from build123d import *

# Parameters (mm, degrees)
SHELL_3_T                 = 2
CUT_EXTRUDE_START         = 8.179460037
CUT_EXTRUDE_8_OUTLINE_W   = 19.681614291
CUT_EXTRUDE_8_OUTLINE_H   = 19.489043198
CUT_EXTRUDE_8_OUTLINE_W_2 = 22.765402734
CUT_EXTRUDE_8_OUTLINE_H_2 = 19.26138917
CUT_EXTRUDE_8_DEPTH       = 11.858295625
SKETCH_9_W                = 37.384578993
SKETCH_9_H                = 19.297136137
CUT_EXTRUDE_5_DEPTH       = 10
CUT_EXTRUDE_10_DEPTH      = 49


# Read off the part's stored shape, not the designer's step: the extrude step
with BuildPart() as part:
    # Sketch 5 → Loft 2 section 0
    with BuildSketch(Plane.XY):
        with BuildLine():
            Line((123.949416554, -29.058070489), (134.559011277, 0.091551442))
            Line((134.559011277, 0.091551442), (59.000774753, -54.400934133))
            Line((59.000774753, -54.400934133), (89.51414806, -54.400934133))
            Line((89.51414806, -54.400934133), (109.519294053, -29.058070489))
            Line((109.519294053, -29.058070489), (123.949416554, -29.058070489))
        make_face()
    # Sketch 2 → Loft 2 section 1
    with BuildSketch(Plane.XY.offset(-30)):
        with BuildLine():
            Line((134.559011277, 0.091551442), (123.949416554, -29.058070489))
            Line((123.949416554, -29.058070489), (109.519294053, -29.058070489))
            Line((109.519294053, -29.058070489), (89.51414806, -54.400934133))
            Line((89.51414806, -54.400934133), (59.000774753, -54.400934133))
            Line((59.000774753, -54.400934133), (134.559011277, 0.091551442))
        make_face()
    loft()

    # Shell 3
    shell_3_openings = [part.faces().sort_by_distance(p)[0] for p in [
        (99.793796859, -32.953132271, 0),
    ]]
    offset(amount=SHELL_3_T, openings=shell_3_openings, kind=Kind.INTERSECTION)

    # Cut-Extrude 8 outline → Cut-Extrude 8 (cut)
    with BuildSketch(Plane(origin=(45.99732156, -63.779004852, 0), x_dir=(0.8110731554347567, 0.5849447294686114, 0), z_dir=(0.5849447294686114, -0.8110731554347567, 0)).offset(CUT_EXTRUDE_START)):
        with Locations((87.31465052, -9.744521599)):
            Rectangle(CUT_EXTRUDE_8_OUTLINE_W, CUT_EXTRUDE_8_OUTLINE_H)
        with Locations((40.58343187, -9.630694585)):
            Rectangle(CUT_EXTRUDE_8_OUTLINE_W_2, CUT_EXTRUDE_8_OUTLINE_H_2)
    extrude(amount=CUT_EXTRUDE_8_DEPTH, mode=Mode.SUBTRACT)

    # Sketch 9 → Cut-Extrude 5 (cut)
    with BuildSketch(Plane(origin=(44.827432101, -62.156858541, 0), x_dir=(0.8110731554347567, 0.5849447294686114, 0), z_dir=(-0.5849447294686114, 0.8110731554347567, 0))):
        with Locations((72.683721601, 9.648568069)):
            Rectangle(SKETCH_9_W, SKETCH_9_H)
    extrude(amount=-CUT_EXTRUDE_5_DEPTH, mode=Mode.SUBTRACT)

    # Sketch 13 → Cut-Extrude 10 (cut)
    with BuildSketch(Plane.XY.offset(-30)):
        Polygon((78.963932985, -44.04826302), (81.023403307, -46.903885112), (89.476536517, -40.807498262), (87.417066196, -37.95187617), align=None)
        Polygon((103.880127445, -22.95550088), (118.225703578, -12.609493132), (121.093195937, -16.585503101), (106.747619804, -26.931510849), align=None)
    extrude(amount=-CUT_EXTRUDE_10_DEPTH, mode=Mode.SUBTRACT)


solid = part.part
Source: CAD feature listing. Evaluate the final solid. Frame: model axes, mm. A direction names the side the tool comes from. Give positions to 0.01 mm unless a question says otherwise; leave off trailing zeros. Write each loop counter-clockwise with the first axis right and the second up, starting at its lowest first coordinate (ties: lowest second). Pieces come first, ordered by that corner, then holes. Notation, with made-up numbers: M 53.5,67 L 88.5,67 A14 ccw 88.5,71 Z; hole C 42,-35.5 d2. An arc over 180 degrees is marked long. Answer as a JSON object with one key per item and string values.
Q1. Cut plane C-C, the plane x = 86.5. Return the cut outline in (y, z).
Geometry check:
{"outline": "M -56.4,-32 L -42.95,-32 L -42.95,-30 L -54.4,-30 L -54.4,-19.26 L -56.4,-19.26 Z; M -38.61,-32 L -32.1,-32 L -32.1,0 L -34.57,0 L -34.57,-30 L -38.61,-30 Z"}
Q2. Cut plane D-D, the plane z = -28.5. Return the cut outline in (x, y).
Geometry check:
{"outline": "M 52.81,-56.4 L 90.48,-56.4 L 110.49,-31.06 L 125.35,-31.06 L 138.66,5.52 Z; hole M 59,-54.4 L 89.51,-54.4 L 109.52,-29.06 L 123.95,-29.06 L 134.56,0.09 Z"}
Q3. Cut plane A-A, the plane z = -1.5. Return the cut outline in (x, y), then the cut area to 3 significant figures.
Geometry check:
{"outline": "M 52.81,-56.4 L 76.68,-56.4 L 75.24,-54.4 L 59,-54.4 L 89.79,-32.2 L 88.62,-30.57 Z; M 96.72,-45.27 L 97.94,-46.96 L 110.49,-31.06 L 117.92,-31.06 L 116.48,-29.06 L 109.52,-29.06 Z; M 118.94,-8.71 L 120.11,-10.33 L 134.56,0.09 L 129.58,-13.58 L 131,-15.54 L 138.66,5.52 Z", "area": "257 mm^2"}
Q4. Contact query for flat-ended pins moving along their axis: P1, Ø19, axis at x = 103, y = -19, coming from the +Z side; P2, Ø4, axis at y = -29, z = -16.5, coming from the -X side; P3, Ø2, axis at x = 121.5, y = -29.5, coming from the +Z side. Output: stop coordinate, or through.
Geometry check:
{"P1": "stops at z = -19.3", "P2": "stops at x = 88.03", "P3": "stops at z = -19.49"}
Q5. Access query for faces 5 (the face through (116, -31.058, -20)), 6 (the face through (105.334, -24.971, -30.986)), 7 (the face through (130.36, -11.45, -18.54)), 8 (the face through (97.32, -46.1, -9.77)), 9 (the face through (117.188, -30.044, -9.881)). Directions: +Z, -Z, +X, -X, +Y, -Y. A direction counts if a zero-diameter tool reaches every point of the face in a straight line with its end or side. Return the directions, or none.
Geometry check:
{"face 5": "+Z, -Z, +X, -Y", "face 6": "+Z, -Z", "face 7": "+Z", "face 8": "+Z, -Y", "face 9": "+Z, +X, +Y"}
Q6. Ray query, line 1 along Y through (x, z) = (62, -27); line 2 along X through (y, z) = (-41.5, -9.5); line 3 along X through (y, z) = (-46.5, -4). Return the intervals inside material, ascending.
Geometry check:
{"line 1": "y = -56.4 to -54.4, -52.24 to -49.77", "line 2": "x = 73.47 to 76.89, 99.7 to 102.25", "line 3": "x = 66.54 to 69.96, 97.61 to 98.3"}
Q7. Cut plane B-B, the plane y = -21.5. Return the cut outline in (x, z), then the cut area to 3 significant figures.
Geometry check:
{"outline": "M 101.2,-32 L 105.9,-32 L 105.9,-30 L 104.62,-30 L 104.62,-19.3 L 101.2,-19.3 Z; M 114.28,-32 L 128.83,-32 L 128.83,-19.49 L 126.7,-19.49 L 126.7,-30 L 114.28,-30 Z", "area": "97.5 mm^2"}
Q8. Mould query, pull axis X, two halves, no side actions, for faces 1 (the face through (101, -33, -30)), 2 (the face through (85.19, -43.9, -30.99)), 3 (the face through (67, -56.401, -16)), 4 (the face through (133.392, -8.963, -19.78)). Classes: +X half, -X half, draft (parallel to the pull), parting line (faces both ways), or undercut.
Geometry check:
{"face 1": "undercut", "face 2": "undercut", "face 3": "draft", "face 4": "+X half"}
